```python
from build123d import *

# Parameters (mm, degrees)
F0_W      = 81.15
F0_H      = 44
F0_R      = 1.65
F0_R_2    = 3
F1_DEPTH  = 8
F2_R      = 17.5
F3_DEPTH  = 2
F4_W      = 33.15
F4_H      = 44
F4_R      = 1.65
F4_R_2    = 7.6
F5_DEPTH  = 2
F6_R      = 6.5
F7_DEPTH  = 3
F8_R      = 7.6
F9_DEPTH  = 2
F10_R     = 6.6
F11_DEPTH = 10
F13_DEPTH = 2
F14_SIZE  = 5


with BuildPart() as f1:
    # F0 (on Front) → F1 (new body)
    with BuildSketch(Plane.XZ):
        with Locations((-172.492545, -67.164728)):
            Rectangle(F0_W, F0_H)
        with Locations((-207.067545, -82.664728)):
            Circle(F0_R, mode=Mode.SUBTRACT)
        with Locations((-176.067545, -82.664728)):
            Circle(F0_R, mode=Mode.SUBTRACT)
        with Locations((-191.567545, -67.164728)):
            Circle(F0_R_2, mode=Mode.SUBTRACT)
        with BuildLine():
            ThreePointArc((-168.067545, -84.237147), (-168.567545, -84.314728), (-169.067545, -84.237147))
            ThreePointArc((-169.067545, -84.237147), (-171.217545, -82.664728), (-169.067545, -81.09231))
            ThreePointArc((-169.067545, -81.09231), (-168.567545, -81.014728), (-168.067545, -81.09231))
            ThreePointArc((-168.067545, -81.09231), (-165.917545, -82.664728), (-168.067545, -84.237147))
        make_face(mode=Mode.SUBTRACT)
        with BuildLine():
            ThreePointArc((-137.067545, -84.237147), (-137.567545, -84.314728), (-138.067545, -84.237147))
            ThreePointArc((-138.067545, -84.237147), (-140.217545, -82.664728), (-138.067545, -81.09231))
            ThreePointArc((-138.067545, -81.09231), (-137.567545, -81.014728), (-137.067545, -81.09231))
            ThreePointArc((-137.067545, -81.09231), (-134.917545, -82.664728), (-137.067545, -84.237147))
        make_face(mode=Mode.SUBTRACT)
        with BuildLine():
            ThreePointArc((-152.567545, -70.122768), (-153.067545, -70.164728), (-153.567545, -70.122768))
            ThreePointArc((-153.567545, -70.122768), (-157.067545, -67.164728), (-153.567545, -64.206688))
            ThreePointArc((-153.567545, -64.206688), (-153.067545, -64.164728), (-152.567545, -64.206688))
            ThreePointArc((-152.567545, -64.206688), (-149.067545, -67.164728), (-152.567545, -70.122768))
        make_face(mode=Mode.SUBTRACT)
        with Locations((-207.067545, -51.664728)):
            Circle(F0_R, mode=Mode.SUBTRACT)
        with Locations((-176.067545, -51.664728)):
            Circle(F0_R, mode=Mode.SUBTRACT)
        with BuildLine():
            ThreePointArc((-168.067545, -53.237147), (-168.567545, -53.314728), (-169.067545, -53.237147))
            ThreePointArc((-169.067545, -53.237147), (-171.217545, -51.664728), (-169.067545, -50.09231))
            ThreePointArc((-169.067545, -50.09231), (-168.567545, -50.014728), (-168.067545, -50.09231))
            ThreePointArc((-168.067545, -50.09231), (-165.917545, -51.664728), (-168.067545, -53.237147))
        make_face(mode=Mode.SUBTRACT)
        with BuildLine():
            ThreePointArc((-137.067545, -53.237147), (-137.567545, -53.314728), (-138.067545, -53.237147))
            ThreePointArc((-138.067545, -53.237147), (-140.217545, -51.664728), (-138.067545, -50.09231))
            ThreePointArc((-138.067545, -50.09231), (-137.567545, -50.014728), (-137.067545, -50.09231))
            ThreePointArc((-137.067545, -50.09231), (-134.917545, -51.664728), (-137.067545, -53.237147))
        make_face(mode=Mode.SUBTRACT)
    extrude(amount=F1_DEPTH)

    # F2 (on face) → F3 (cut)
    with BuildSketch(Plane(origin=(0, 0, 0), x_dir=(-1, 0, 0), z_dir=(0, 1, 0))):
        with Locations((153.067545, -67.164728)):
            Circle(F2_R)
    extrude(amount=-F3_DEPTH, mode=Mode.SUBTRACT)

    # F4 (on face) → F5 (join)
    with BuildSketch(Plane(origin=(0, 0, 0), x_dir=(-1, 0, 0), z_dir=(0, 1, 0))):
        with Locations((196.492545, -67.164728)):
            Rectangle(F4_W, F4_H)
        with Locations((207.067545, -82.664728)):
            Circle(F4_R, mode=Mode.SUBTRACT)
        with Locations((191.567545, -67.164728)):
            Circle(F4_R_2, mode=Mode.SUBTRACT)
        with Locations((207.067545, -51.664728)):
            Circle(F4_R, mode=Mode.SUBTRACT)
    extrude(amount=F5_DEPTH)

    # F6 (on face) → F7 (cut)
    with BuildSketch(Plane(origin=(0, 2, 0), x_dir=(-1, 0, 0), z_dir=(0, 1, 0))):
        with Locations((191.567545, -67.164728)):
            Circle(F6_R)
    extrude(amount=-F7_DEPTH, mode=Mode.SUBTRACT)

    # F8 (on face) → F9 (cut)
    with BuildSketch(Plane.XZ.offset(8)):
        with Locations((-191.567545, -67.164728)):
            Circle(F8_R)
    extrude(amount=-F9_DEPTH, mode=Mode.SUBTRACT)

    # F10 (on face) → F11 (cut)
    with BuildSketch(Plane.XZ.offset(8)):
        with Locations((-191.567545, -67.164728)):
            Circle(F10_R)
    extrude(amount=-F11_DEPTH, mode=Mode.SUBTRACT)

    # F12 (on face) → F13 (join)
    with BuildSketch(Plane(origin=(0, 0, 0), x_dir=(-1, 0, 0), z_dir=(0, 1, 0))):
        with BuildLine():
            ThreePointArc((176.067545, -81.064728), (177.667545, -82.664728), (176.067545, -84.264728))
            Line((176.067545, -84.264728), (176.067545, -85.664728))
            Line((176.067545, -85.664728), (179.917545, -85.664728))
            Line((179.917545, -85.664728), (179.917545, -79.664728))
            Line((179.917545, -79.664728), (176.067545, -79.664728))
            Line((176.067545, -79.664728), (176.067545, -81.064728))
        make_face()
        with BuildLine():
            Line((176.067545, -53.264728), (176.067545, -54.664728))
            Line((176.067545, -54.664728), (179.917545, -54.664728))
            Line((179.917545, -54.664728), (179.917545, -48.664728))
            Line((179.917545, -48.664728), (176.067545, -48.664728))
            Line((176.067545, -48.664728), (176.067545, -50.064728))
            ThreePointArc((176.067545, -50.064728), (177.667545, -51.664728), (176.067545, -53.264728))
        make_face()
    extrude(amount=F13_DEPTH)

    # F14
    f14_edges = [f1.edges().sort_by_distance(p)[0] for p in [
        (-213.067545, -3, -89.164728),
        (-213.067545, -3, -45.164728),
        (-131.917545, -4, -89.164728),
        (-131.917545, -4, -45.164728),
    ]]
    chamfer(f14_edges, length=F14_SIZE)


solid = f1.part
```
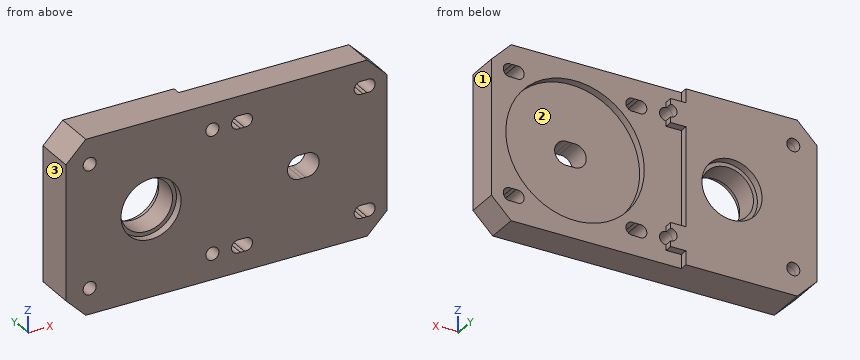
Can you work these out from the model? Positions are in its coordinate system, mm. Face numbers are marked on the shaded views. Coordinates: 2 decimals unless noted, no trailing zeros. Loops run counter-clockwise (first coordinate to the right, second up) from the corner with the lowest first, then second, coordinate; pieces in that order, holes last. Notation, with made-up numbers: (37, 41.5) -> (94, 41.5) arc R21 ccw to (94, 57.5) -> close; hole circle Ø6 at (89, 72.5). An arc over 180 degrees is marked (long way). Put each result on its own line as item: value. Start each with the question number.
Q1. I want a section at B-B (y = -2.75). Count the separate pieces of the cut face and the enclosed holes in it, plus the area to 3 significant figures.
Q2. I'm going to push flat-ended pins straight in: P1, Ø13.5, axis at x = -191.57, z = -67.16, coming from the -Y side; P2, Ø1, axis at x = -177, y = 1, coming from the -Z side; P3, Ø4.5, axis at x = -207.07, z = -51.66, coming from the +Y side; P4, Ø3, axis at x = -167.57, z = -51.66, coming from the +Y side. Where does each tip first touch, or does it pass through?
Q3. I want a section at A-A (z = -68.5). Write out the boundary of the cut face in (x, y).
Q4. If I drill on line 1 (Z direction, x = -176, y = -4); line 2 (Z direction, x = -168, y = -3.25); line 3 (X direction, y = -2.75, z = -64.5), over which ranges is the centre line in solid material (lowest first)? Write a range as [from, to].
Q5. I want a section at D-D (y = 1.25). Write out the boundary of the cut face in (x, z).
Q6. Thinking about a two-plate mould opening in X: for the marked faces 1, 2 and 3, which applies, pulls with the +X half, pulls with the -X half, needs draft (parallel to the pull), parting line crosses it, or undercut?
Q7. I want a section at C-C (x = -155.5). Write out the boundary of the cut face in (y, z).
Taken from the geometry:
1. separate pieces: 1
1. enclosed holes: 10
1. area: 3,250 mm2
2. P1: stops at y = -6
2. P2: stops at z = -85.66
2. P3: stops at y = 2
2. P4: passes through
3. outline: (-213.07, -8) -> (-199.05, -8) -> (-199.05, -6) -> (-198.03, -6) -> (-198.03, 0) -> (-199.05, 0) -> (-199.05, 2) -> (-213.07, 2) -> close; (-185.1, -6) -> (-184.09, -6) -> (-184.09, -8) -> (-156.75, -8) -> (-156.75, -2) -> (-170.52, -2) -> (-170.52, 0) -> (-179.92, 0) -> (-179.92, 2) -> (-184.09, 2) -> (-184.09, 0) -> (-185.1, 0) -> close; (-149.38, -8) -> (-131.92, -8) -> (-131.92, 0) -> (-135.62, 0) -> (-135.62, -2) -> (-149.38, -2) -> close
4. line 1: z = [-89.16, -84.31], [-81.02, -53.31], [-50.02, -45.16]
4. line 2: z = [-89.16, -84.26], [-81.07, -53.26], [-50.07, -45.16]
4. line 3: x = [-213.07, -197.61], [-185.53, -155.45], [-150.69, -131.92]
5. outline: (-213.07, -84.16) -> (-208.07, -89.16) -> (-179.92, -89.16) -> (-179.92, -85.66) -> (-176.07, -85.66) -> (-176.07, -84.26) arc R1.6 cw to (-176.07, -81.06) -> (-176.07, -79.66) -> (-179.92, -79.66) -> (-179.92, -54.66) -> (-176.07, -54.66) -> (-176.07, -53.26) arc R1.6 cw to (-176.07, -50.06) -> (-176.07, -48.66) -> (-179.92, -48.66) -> (-179.92, -45.16) -> (-208.07, -45.16) -> (-213.07, -50.16) -> close; hole circle Ø3.3 at (-207.07, -82.66); hole circle Ø3.3 at (-207.07, -51.66); hole circle Ø15.2 at (-191.57, -67.16)
6. face 1: pulls with the +X half
6. face 2: undercut
6. face 3: pulls with the -X half
7. outline: (-8, -89.16) -> (0, -89.16) -> (0, -84.49) -> (-2, -84.49) -> (-2, -69.8) -> (-8, -69.8) -> close; (-8, -64.53) -> (-2, -64.53) -> (-2, -49.83) -> (0, -49.83) -> (0, -45.16) -> (-8, -45.16) -> close
